```python
from build123d import *

# Parameters (mm, degrees)
SKETCH1_W                = 78.58
SKETCH1_H                = 52.04
BOSS_EXTRUDE1_DEPTH      = 0.7
EDGE_FLANGE2_DEPTH       = 52.04
EDGE_FLANGE1_START       = -39.29
EDGE_FLANGE1_DEPTH       = 78.58
EDGE_FLANGE1_START_2     = -40.75
EDGE_FLANGE1_2_OUTLINE_W = 18.34
EDGE_FLANGE1_2_OUTLINE_H = 0.7
EDGE_FLANGE1_2_DEPTH     = 81.5
CUT_EXTRUDE1_REACH       = 90.258
SKETCH12_W               = 3
SKETCH12_H               = 10
LPATTERN1_COUNT          = 7
LPATTERN1_PITCH          = 6
SKETCH13_W               = 3
SKETCH13_H               = 10
CUT_EXTRUDE2_DEPTH       = 88.611816555
CUT_EXTRUDE3_REACH       = 90.258
SKETCH14_W               = 19
SKETCH14_H               = 10.5
SKETCH15_W               = 0.7
SKETCH15_H               = 1.6
BOSS_EXTRUDE2_DEPTH      = 2.3
CUT_EXTRUDE4_REACH       = 73.877
SKETCH16_W               = 67
SKETCH16_H               = 11.5
SKETCH17_W               = 27.5
SKETCH17_H               = 0.7
BOSS_EXTRUDE3_DEPTH      = 1.8
M3_CLEARANCE_HOLE2_D     = 3.4


# Read off the part's stored shape, not the designer's step: Edge-Flange1
# Sheet-metal steps are written as plain solids
with BuildPart() as part:
    # Sketch1 → Boss-Extrude1 (new body)
    with BuildSketch(Plane(origin=(0, 0, 0), x_dir=(1, 0, 0), z_dir=(0, 1, 0))):
        Rectangle(SKETCH1_W, SKETCH1_H)
    extrude(amount=-BOSS_EXTRUDE1_DEPTH)

    # Edge-Flange2 section (across the edge) → Edge-Flange2 (add)
    with BuildSketch(Plane(origin=(40.05, -0.7, -26.02), x_dir=(-1, 0, 0), z_dir=(0, 0, 1))):
        with BuildLine():
            Line((-0.7, 0.76), (-0.7, 19.1))
            Line((-0.7, 19.1), (0, 19.1))
            Line((0, 19.1), (0, 0.76))
            ThreePointArc((0, 0.76), (0.222598846, 0.222598846), (0.76, 0))
            Line((0.76, 0), (0.76, -0.7))
            ThreePointArc((0.76, -0.7), (-0.272375901, -0.272375901), (-0.7, 0.76))
        make_face()
    edge_flange2 = extrude(amount=EDGE_FLANGE2_DEPTH)

    # Mirror1: Edge-Flange2 across plane
    add(edge_flange2.mirror(Plane(origin=(0, 0, 0), x_dir=(0, 0, 1), z_dir=(1, 0, 0))))

    # Edge-Flange1 outline → Edge-Flange1 (add)
    with BuildSketch(Plane.YZ.offset(EDGE_FLANGE1_START)):
        with BuildLine():
            Line((-1.46, 27.48), (-19.8, 27.48))
            Line((-19.8, 27.48), (-19.8, 26.78))
            Line((-19.8, 26.78), (-1.46, 26.78))
            ThreePointArc((-1.46, 26.78), (-0.922598846, 26.557401154), (-0.7, 26.02))
            Line((-0.7, 26.02), (0, 26.02))
            ThreePointArc((0, 26.02), (-0.427624099, 27.052375901), (-1.46, 27.48))
        make_face()
    extrude(amount=EDGE_FLANGE1_DEPTH)

    # Edge-Flange1 2 outline → Edge-Flange1 2 (add)
    with BuildSketch(Plane.YZ.offset(EDGE_FLANGE1_START_2)):
        with Locations((-10.63, 27.13)):
            Rectangle(EDGE_FLANGE1_2_OUTLINE_W, EDGE_FLANGE1_2_OUTLINE_H)
    extrude(amount=EDGE_FLANGE1_2_DEPTH)

    # Sketch12 → Cut-Extrude1 (cut, up to next)
    with BuildSketch(Plane.ZY.offset(40.75), mode=Mode.PRIVATE) as cut_extrude1_sk1:
        with Locations((-17.02, -10.3)):
            Rectangle(SKETCH12_W, SKETCH12_H)
    cut_extrude1_tool1 = extrude(cut_extrude1_sk1.sketch, amount=-CUT_EXTRUDE1_REACH, mode=Mode.PRIVATE) & part.part
    cut_extrude1 = cut_extrude1_tool1.solids().sort_by_distance((-40.75, -10.3, -17.02))[0]
    add(cut_extrude1, mode=Mode.SUBTRACT)

    # LPattern1: Cut-Extrude1 ×7
    with Locations(*[(0, 0, i * LPATTERN1_PITCH) for i in range(1, LPATTERN1_COUNT)]):
        add(cut_extrude1, mode=Mode.SUBTRACT)

    # Sketch13 → Cut-Extrude2 (cut, through all)
    with BuildSketch(Plane.ZY.offset(-40.05)):
        with Locations((18.98, -10.3)):
            Rectangle(SKETCH13_W, SKETCH13_H)
        with Locations((-11.02, -10.3)):
            Rectangle(SKETCH13_W, SKETCH13_H)
        with Locations((-17.02, -10.3)):
            Rectangle(SKETCH13_W, SKETCH13_H)
    extrude(amount=-CUT_EXTRUDE2_DEPTH, mode=Mode.SUBTRACT)

    # Sketch14 → Cut-Extrude3 (cut, up to next)
    with BuildSketch(Plane(origin=(40.75, 0, 0), x_dir=(0, 0, -1), z_dir=(1, 0, 0)), mode=Mode.PRIVATE) as cut_extrude3_sk1:
        with Locations((-2.48, -8.25)):
            Rectangle(SKETCH14_W, SKETCH14_H)
    cut_extrude3_tool1 = extrude(cut_extrude3_sk1.sketch, amount=-CUT_EXTRUDE3_REACH, mode=Mode.PRIVATE) & part.part
    add(cut_extrude3_tool1.solids().sort_by_distance((40.75, -8.25, 2.48))[0], mode=Mode.SUBTRACT)

    # Sketch15 → Boss-Extrude2 (add)
    with BuildSketch(Plane(origin=(0, 0, -26.02), x_dir=(-1, 0, 0), z_dir=(0, 0, -1))):
        with Locations((-40.4, -5.9)):
            Rectangle(SKETCH15_W, SKETCH15_H)
    boss_extrude2 = extrude(amount=BOSS_EXTRUDE2_DEPTH)

    # Mirror2: Boss-Extrude2 across plane
    add(boss_extrude2.mirror(Plane(origin=(0, 0, 0), x_dir=(0, 0, 1), z_dir=(1, 0, 0))))

    # Sketch16 → Cut-Extrude4 (cut, up to next)
    with BuildSketch(Plane.XY.offset(27.48), mode=Mode.PRIVATE) as cut_extrude4_sk1:
        with Locations((0.45, -8.25)):
            Rectangle(SKETCH16_W, SKETCH16_H)
    cut_extrude4_tool1 = extrude(cut_extrude4_sk1.sketch, amount=-CUT_EXTRUDE4_REACH, mode=Mode.PRIVATE) & part.part
    add(cut_extrude4_tool1.solids().sort_by_distance((0.45, -8.25, 27.48))[0], mode=Mode.SUBTRACT)

    # Sketch17 → Boss-Extrude3 (add)
    with BuildSketch(Plane(origin=(0, 0, -26.02), x_dir=(-1, 0, 0), z_dir=(0, 0, -1))):
        with Locations((0, -0.35)):
            Rectangle(SKETCH17_W, SKETCH17_H)
    extrude(amount=BOSS_EXTRUDE3_DEPTH)

    # M3 Clearance Hole2 (through all)
    with Locations(Plane(origin=(0, 0, 0), x_dir=(1, 0, 0), z_dir=(0, 1, 0))):
        with Locations((34.3, -16.98)):
            m3_clearance_hole2 = Hole(M3_CLEARANCE_HOLE2_D / 2)

    # Mirror3: M3 Clearance Hole2 across plane
    add(m3_clearance_hole2.mirror(Plane(origin=(0, 0, 0), x_dir=(0, 0, 1), z_dir=(1, 0, 0))), mode=Mode.SUBTRACT)


solid = part.part
```
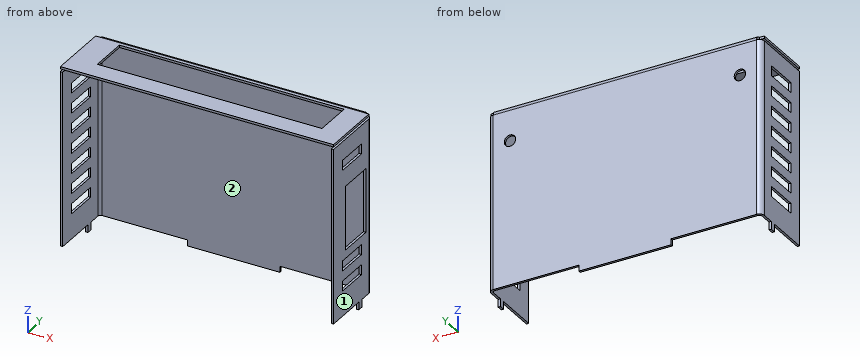
Read the model definition and answer for the solid it produces. Units are mm, in the model's axes. Face numbers are marked on the shaded views. A direction names the side the tool comes from. Round coordinates to 2 decimals unless told otherwise and drop trailing zeros. Write each loop counter-clockwise with the first axis right and the second up, starting at its lowest first coordinate (ties: lowest second). Pieces come first, ordered by that corner, then holes. Notation, with made-up numbers: M -16,0 L 37,0 A20 cw 37,39 Z; hole C 50,42.25 d9. An arc over 180 degrees is marked long. One line per item, written item: value.
Q1. Find section D-D on y = -11.75. Count the separate pieces of the cut face and the enclosed holes in it, plus the area to 3 significant figures.
Data:
separate pieces: 15
enclosed holes: 0
area: 48.7 mm2
Q2. Which of the six approach directions +Z, -Z, +X, -X, +Y, -Y give full straight-line access (tool end or side, diameter ignored) to the marked faces 1 and 2?
Data:
face 1: +Z, -Z, +X, +Y, -Y
face 2: -Z, -Y
Q3. Find section B-B on z = -17. Write down the section's boundary in (x, y).
Data:
outline: M -40.75,-19.8 L -40.05,-19.8 L -40.05,-15.3 L -40.75,-15.3 Z; M -40.75,-5.3 L -40.05,-5.3 L -40.05,-1.46 A0.76 cw -39.29,-0.7 L 39.29,-0.7 A0.76 cw 40.05,-1.46 L 40.05,-5.3 L 40.75,-5.3 L 40.75,-1.46 A1.46 ccw 39.29,0 L -39.29,0 A1.46 ccw -40.75,-1.46 Z; M 40.05,-19.8 L 40.75,-19.8 L 40.75,-15.3 L 40.05,-15.3 Z
Q4. Straight lines are drawn through the part: line 1 (X direction, y = -17, z = -25); line 2 (Y direction, x = -33, z = 24); line 3 (Z direction, x = 34, y = -13.25). For each, find the intervals that lie inside material, in ascending order. Write a range as [from, to].
Data:
line 1: [-40.75, -40.05], [40.05, 40.75]
line 2: [-0.7, 0]
line 3: [26.78, 27.48]
Q5. Flat-ended cylindrical pins translate along their axes: pin 1 Ø1 at (x, y) = (-4.5, -4.5) entering from +Z; pin 2 Ø12 at (x, z) = (-24.5, -2.5) entering from -Y; pin 3 Ø4 at (x, y) = (22.5, -3.5) entering from -Z; pin 4 Ø0.8 at (x, y) = (-40.5, -8.5) entering from -Z. Find the tip coordinate at first contact, or state that the pin passes through.
Data:
pin 1: through
pin 2: y = -0.7
pin 3: z = 26.78
pin 4: z = -26.02
Q6. Find section A-A on x = -11.5. Write down the section's boundary in (y, z).
Data:
outline: M -19.8,26.78 L -14,26.78 L -14,27.48 L -19.8,27.48 Z; M -2.5,26.78 L -1.46,26.78 A0.76 cw -0.7,26.02 L -0.7,-27.82 L 0,-27.82 L 0,26.02 A1.46 ccw -1.46,27.48 L -2.5,27.48 Z
Q7. Find section C-C on x = -34.3. Write down the section's boundary in (y, z).
Data:
outline: M -19.8,26.78 L -1.46,26.78 A0.76 cw -0.7,26.02 L -0.7,18.68 L 0,18.68 L 0,26.02 A1.46 ccw -1.46,27.48 L -19.8,27.48 Z; M -0.7,-26.02 L 0,-26.02 L 0,15.28 L -0.7,15.28 Z
